Read the model definition and answer for the solid it produces. Units are mm, in the model's axes. A direction names the side the tool comes from. Give positions to 0.01 mm unless a question says otherwise; leave off trailing zeros. Write each loop counter-clockwise with the first axis right and the second up, starting at its lowest first coordinate (ties: lowest second). Pieces come first, ordered by that corner, then holes. Notation, with made-up numbers: (84, 22) - (143, 22) arc R14 cw to (143, 37) - close; hole circle Ø3 at (-15.75, 62). An arc over 180 degrees is marked (long way). Answer as CSV lines item,"result".
```python
from build123d import *

# Parameters (mm, degrees)
EXTRUDE_1_DEPTH     = 5
SKETCH_2_R          = 5.000000000012101
EXTRUDE_3_DEPTH     = 27.5
CUT_EXTRUDE_1_DEPTH = 59.80000000000002
SKETCH_4_R          = 5.0000000000065405
SKETCH_4_R_2        = 5.000000000006525
EXTRUDE_4_DEPTH     = 12
CUT_EXTRUDE_2_DEPTH = 39.00000000000001
FILLET_1_R          = 2


with BuildPart() as part:
    # 草图1 → 凸台-拉伸1 (new body)
    with BuildSketch(Plane(origin=(-35.95282664063733, 399.74242683802464, 30.566209896758863), x_dir=(0.9960030029050825, 0.08905977205298914, 0.006809934355634975), z_dir=(-0.0893197525973871, 0.9931039643902259, 0.07593745919082788))):
        with BuildLine():
            Line((300.07791562372654, -1129.6042951871439), (302.10510848643986, -1072.2401034897346))
            Line((302.10510848643986, -1072.2401034897346), (327.3060115945207, -1073.1306780695022))
            ThreePointArc((327.3060115945207, -1073.1306780695022), (330.1251349541227, -1073.6036481637962), (332.72578534648983, -1074.7901450088955))
            Line((332.72578534648983, -1074.7901450088955), (351.6029613751, -1086.5968806615322))
            ThreePointArc((351.6029613751, -1086.5968806615322), (355.4148735940491, -1088.3359924755819), (359.5470133129178, -1089.029250011054))
            Line((359.5470133129178, -1089.029250011054), (465.98440043114425, -1092.7906402635294))
            ThreePointArc((465.98440043114425, -1092.7906402635294), (470.1551691567732, -1092.390799165044), (474.0803358930331, -1090.9251079426926))
            Line((474.0803358930331, -1090.9251079426926), (493.74385691829394, -1080.480361776527))
            ThreePointArc((493.74385691829394, -1080.480361776527), (496.42177441125835, -1079.4804042136147), (499.26725213995996, -1079.2076154267972))
            Line((499.26725213995996, -1079.2076154267972), (497.24005927724687, -1136.5718071242063))
            ThreePointArc((497.24005927724687, -1136.5718071242063), (494.4209359176449, -1136.0988370299121), (491.8202855252778, -1134.9123401848128))
            Line((491.8202855252778, -1134.9123401848128), (472.9431094966676, -1123.1056045321764))
            ThreePointArc((472.9431094966676, -1123.1056045321764), (469.13119727771857, -1121.3664927181267), (464.9990575588499, -1120.6732351826547))
            Line((464.9990575588499, -1120.6732351826547), (358.5616704406234, -1116.9118449301766))
            ThreePointArc((358.5616704406234, -1116.9118449301766), (354.39090171499237, -1117.3116860286625), (350.4657349787294, -1118.777377251013))
            Line((350.4657349787294, -1118.777377251013), (330.80221395347337, -1129.222123417182))
            ThreePointArc((330.80221395347337, -1129.222123417182), (328.12429646050896, -1130.2220809800938), (325.2788187318076, -1130.494869766911))
            Line((325.2788187318076, -1130.494869766911), (300.07791562372654, -1129.6042951871439))
        make_face()
    extrude(amount=-EXTRUDE_1_DEPTH)

    # 草图2 → 凸台-拉伸3 (add, symmetric)
    with BuildSketch(Plane(origin=(-38.327599823670674, -86.44895602357099, 1085.4904824160742), x_dir=(0.9993811405079088, -0.0027925735986703876, 0.03506476193855483), z_dir=(-0.03517578708588501, -0.07933995566829466, 0.9962267991965693))):
        with Locations((318.1419856303242, 426.65964110326615)):
            Circle(SKETCH_2_R)
    extrude(amount=EXTRUDE_3_DEPTH, both=True)

    # 草图3 → 切除-拉伸1 (cut)
    with BuildSketch(Plane(origin=(-39.33714491302575, -88.72601275125034, 1114.0821915530184), x_dir=(0.9993811405079092, -0.002792573598669658, 0.03506476193854602), z_dir=(-0.03517578708587617, -0.07933995566829388, 0.9962267991965696))):
        Polygon((321.1034402768945, 426.9253847947825), (319.3925721658551, 429.35720790511795), (316.43111751927484, 429.0914642136009), (315.18053098373395, 426.39389741174824), (316.8913990947733, 423.9620743014128), (319.8528537413536, 424.2278179929299), align=None)
    extrude(amount=-CUT_EXTRUDE_1_DEPTH, mode=Mode.SUBTRACT)

    # 草图4 → 凸台-拉伸4 (add, symmetric)
    with BuildSketch(Plane(origin=(-38.327599823670674, -86.44895602357099, 1085.4904824160742), x_dir=(0.9993811405079088, -0.0027925735986703876, 0.03506476193855483), z_dir=(-0.03517578708588501, -0.07933995566829466, 0.9962267991965693))):
        with Locations((368.7211342547294, 431.1983193115499)):
            Circle(SKETCH_4_R)
        with Locations((458.86276991896267, 439.2871046820992)):
            Circle(SKETCH_4_R_2)
    extrude(amount=EXTRUDE_4_DEPTH, both=True)

    # 草图5 → 切除-拉伸2 (cut)
    with BuildSketch(Plane(origin=(-38.81830205352909, -87.55574840514421, 1099.3878462648613), x_dir=(0.9993811405079085, -0.002792573598671172, 0.0350647619385643), z_dir=(-0.035175787085894514, -0.07933995566829542, 0.9962267991965689))):
        Polygon((369.9717207902861, 433.8958861133999), (367.01026614370573, 433.6301424218828), (365.75967960816484, 430.9325756200302), (367.47054771920426, 428.5007525096948), (370.4320023657846, 428.7664962012118), (371.6825889013256, 431.46406300306455), align=None)
        Polygon((460.1133564545191, 441.9846714839496), (457.1519018079389, 441.7189277924325), (455.90131527239805, 439.02136099058004), (457.61218338343764, 436.58953788024445), (460.57363803001766, 436.8552815717618), (461.82422456555855, 439.5528483736145), align=None)
    extrude(amount=-CUT_EXTRUDE_2_DEPTH, mode=Mode.SUBTRACT)

    # 圆角1
    fillet_1_edges = [part.edges().sort_by_distance(p)[0] for p in [
        (415.285524437343, 350.7404864262651, 1136.3250812261313),
        (425.0382330865837, 351.5861636609777, 1136.7367898828338),
        (325.19967377997307, 342.9289587973129, 1132.5221249504996),
        (334.952382429214, 343.7746360320256, 1132.9338336072021),
        (274.6518265417908, 338.545851989709, 1130.3882576287017),
        (284.4045351910414, 339.3915292244225, 1130.7999662854045),
    ]]
    fillet(fillet_1_edges, radius=FILLET_1_R)

    # 切除-扫描1: sweep along a curve in space
    with BuildLine() as sweep_1_path:
        Line((290.044943776391, 347.0743828700847, 1102.8022885042362), (264.94476860482246, 344.89789554811915, 1101.7426895995065))
        ThreePointArc((295.44305470841834, 347.43054527632216, 1104.493833582377), (292.8527991081144, 347.28939307381154, 1103.2930799825197), (290.044943776391, 347.0743828700847, 1102.8022885042362))
        Line((314.24477871928195, 348.21157078080637, 1116.3947560242318), (295.44305470841834, 347.43054527632216, 1104.493833582377))
        ThreePointArc((322.1570783045824, 348.73361704748316, 1118.8741440154793), (318.0414547361659, 348.4184651050343, 1118.1547647253926), (314.24477871928195, 348.21157078080637, 1116.3947560242318))
        Line((428.16903549570674, 357.926129817856, 1123.34941771218), (322.1570783045824, 348.73361704748316, 1118.8741440154793))
        ThreePointArc((436.23261152707437, 358.7893842711662, 1121.5444481339446), (432.32313367085544, 358.32806229446095, 1122.979143081403), (428.16903549570674, 357.926129817856, 1123.34941771218))
        Line((455.8175375159207, 361.33694338754674, 1111.264010490222), (436.23261152707437, 358.7893842711662, 1121.5444481339446))
        ThreePointArc((461.31885574293176, 361.925892687469, 1110.0325826471264), (458.4847513804454, 361.6516770725888, 1110.2851999185907), (455.8175375159207, 361.33694338754674, 1111.264010490222))
    # 草图8 → 切除-扫描1 (sweep, cut)
    with BuildSketch(Plane(origin=(534.589737117881, 46.35536514533573, 22.567599471235773), x_dir=(0.04186275100976178, 0.0036300044207879887, -0.9991167765310519), z_dir=(0.9953816583596613, 0.08631157133878511, 0.042019838816923734))):
        Polygon((-1088.4263068343075, 320.7205078186499), (-1088.5260175810986, 320.71290735982717), (-1088.145994639964, 315.7273700202607), (-1088.046283893173, 315.7349704790834), align=None)
    sweep_1 = sweep(path=sweep_1_path.line, mode=Mode.SUBTRACT)

    # 镜向2: 切除-扫描1 across plane
    add(sweep_1.mirror(Plane(origin=(-38.327599823670674, -86.44895602357099, 1085.4904824160742), x_dir=(0.9993811405079088, -0.002792573598670388, 0.035064761938554824), z_dir=(-0.035175787085885, -0.07933995566829465, 0.9962267991965692))), mode=Mode.SUBTRACT)

    # 镜向3: part across plane


with BuildPart() as part_1:
    add(part.part)
    add(part.part.mirror(Plane(origin=(-38.327599823670674, -86.44895602357099, 1085.4904824160742), x_dir=(0.9993811405079088, -0.002792573598670388, 0.035064761938554824), z_dir=(-0.035175787085885, -0.07933995566829465, 0.9962267991965692))))


solid = part_1.part
```
(1) Each of these flat-tipped pins is pushed along its axis until it touches: P1, Ø12, axis at y = 334.5, z = 1134.5, coming from the +X side; P2, Ø8, axis at x = 322.5, z = 1149.5, coming from the -Y side; P3, Ø4, axis at x = 368, z = 1143, coming from the +Y side. Where does it stop, or does it pass through?
Worked out:
P1,"stops at x = 334.8"
P2,"stops at y = 341.44"
P3,"stops at y = 351.25"
(2) A cutting plane is placed at A-A (x = 362.5). Write down the section's boundary in (y, z).
Worked out:
outline,"(345.11, 1147.92) - (347.22, 1120.28) - (352.22, 1120.68) - (350.11, 1148.31) - close"
(3) A cutting plane is placed at B-B (z = 1139). Count the separate pieces of the cut face and the enclosed holes in it, and give its area (3 significant figures).
Worked out:
separate pieces,"1"
enclosed holes,"3"
area,"1,070 mm^2"
(4) A cutting plane is placed at C-C (x = 440.5). Write down the section's boundary in (y, z).
Worked out:
outline,"(351.48, 1156.26) - (354.31, 1119.27) - (359.34, 1119.42) - (356.47, 1156.92) - close"
(5) Find the intervals of material crossed by L1, parallel to Y at x = 301, z = 1154.5; L2, parallel to Y at x = 385, z = 1146.5; L3, parallel to X at y = 344, z = 1109.5, in increasing order.
Worked out:
L1,"y = 339.07 to 344.11"
L2,"y = 347.24 to 352.27"
L3,"x = 264.7 to 303.96"
(6) For faces 4 (the flat face through (330.369, 339.786, 1132.623)), 5 (the flat face through (332.275, 343.797, 1133.036)), 6 (the flat face through (460.544, 357.233, 1138.038)), determine the directions among +Z, -Z, +X, -X, +Y, -Y from which every point of the face is accessible in a straight line to the end or side of a thin tool.
Worked out:
face 4,"+Z"
face 5,"-Z"
face 6,"+Z, +X, +Y"
(7) The mould has two halves that part along Y. Classify faces 1 (the flat face through (420.035, 352.714, 1136.845)), 2 (the cylindrical face through (432.63, 355.81, 1122.87)), 3 (the cylindrical face through (431.615, 353.524, 1151.594)): +Y half, -Y half, draft (parallel to the pull), parting line (faces both ways), or undercut.
Worked out:
face 1,"undercut"
face 2,"+Y half"
face 3,"-Y half"
